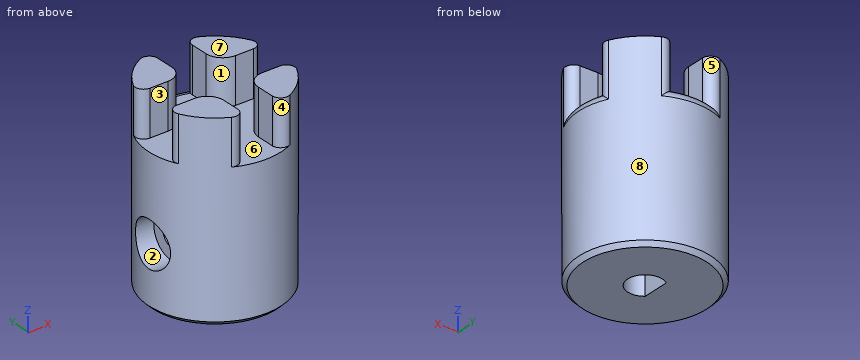
from build123d import *

# Parameters (mm, degrees)
SKETCH1_R           = 8
BOSS_EXTRUDE1_DEPTH = 23
CUT_EXTRUDE1_DEPTH  = 5.5
CHAMFER1_SIZE       = 0.5
FILLET1_R           = 1
SKETCH3_R           = 2.75
CUT_EXTRUDE2_DEPTH  = 15.5
SKETCH5_R           = 3.239790556
SKETCH5_R_2         = 1.3
BOSS_EXTRUDE2_DEPTH = 4


with BuildPart() as part:
    # Sketch1 → Boss-Extrude1 (new body)
    with BuildSketch(Plane.XY):
        Circle(SKETCH1_R)
        with BuildLine():
            Line((-1.3, 1.64924225), (-1.3, -1.64924225))
            ThreePointArc((-1.3, -1.64924225), (2.1, 0), (-1.3, 1.64924225))
        make_face(mode=Mode.SUBTRACT)
    extrude(amount=BOSS_EXTRUDE1_DEPTH)

    # Sketch2 → Cut-Extrude1 (cut)
    with BuildSketch(Plane.XY.offset(23)):
        with BuildLine():
            Line((4.1, 2.1), (9.874781321, 2.1))
            Line((9.874781321, 2.1), (9.874781321, -2.1))
            Line((9.874781321, -2.1), (4.1, -2.1))
            ThreePointArc((4.1, -2.1), (2.685786438, -2.685786438), (2.1, -4.1))
            Line((2.1, -4.1), (2.1, -8.269913673))
            Line((2.1, -8.269913673), (-2.1, -8.269913673))
            Line((-2.1, -8.269913673), (-2.1, -4.1))
            ThreePointArc((-2.1, -4.1), (-2.685786438, -2.685786438), (-4.1, -2.1))
            Line((-4.1, -2.1), (-9.874781321, -2.1))
            Line((-9.874781321, -2.1), (-9.874781321, 2.1))
            Line((-9.874781321, 2.1), (-4.1, 2.1))
            ThreePointArc((-4.1, 2.1), (-2.685786438, 2.685786438), (-2.1, 4.1))
            Line((-2.1, 4.1), (-2.1, 8.269913673))
            Line((-2.1, 8.269913673), (2.1, 8.269913673))
            Line((2.1, 8.269913673), (2.1, 4.1))
            ThreePointArc((2.1, 4.1), (2.685786438, 2.685786438), (4.1, 2.1))
        make_face()
    extrude(amount=-CUT_EXTRUDE1_DEPTH, mode=Mode.SUBTRACT)

    # Chamfer1
    chamfer1_edges = [part.edges().sort_by_distance(p)[0] for p in [
        (-8, 0, 0),
    ]]
    chamfer(chamfer1_edges, length=CHAMFER1_SIZE)

    # Fillet1
    # the kernel refuses this fillet: 1 mm, written as the material it takes off along each edge
    with BuildSketch(Plane(origin=(-7.719455939, 2.1, 26.857409903), x_dir=(0.35433001139154063, 0.9351204430592194, 0), z_dir=(0, 0, -1)), Plane(origin=(-2.1, -7.719455939, 26.857409903), x_dir=(-0.9351204430592192, 0.354330011391541, 0), z_dir=(0, 0, -1)), Plane(origin=(7.719455939, -2.1, 26.857409903), x_dir=(-0.354330011391541, -0.9351204430592192, 0), z_dir=(0, 0, -1)), Plane(origin=(2.1, 7.719455939, 26.857409903), x_dir=(0.935120443059219, -0.3543300113915411, 0), z_dir=(0, 0, -1))) as fillet1_piece_1:
        with BuildLine():
            CenterArc((1.446528713, 0.99533926), FILLET1_R, 159.247612079, 116.286320683)
            Line((0.51140827, 1.349669272), (0, 0))
            ThreePointArc((0, 0), (0.771481981, -0.037285918), (1.542963961, 0))
        make_face()
    extrude(amount=9.357409903, mode=Mode.SUBTRACT)
    with BuildSketch(Plane(origin=(-7.719455939, -2.1, 26.857409903), x_dir=(0.35433001139154124, -0.9351204430592192, 0), z_dir=(0, 0, -1)), Plane(origin=(2.1, -7.719455939, 26.857409903), x_dir=(0.935120443059219, 0.3543300113915412, 0), z_dir=(0, 0, -1)), Plane(origin=(7.719455939, 2.1, 26.857409903), x_dir=(-0.3543300113915409, 0.9351204430592193, 0), z_dir=(0, 0, -1)), Plane(origin=(-2.1, 7.719455939, 26.857409903), x_dir=(-0.935120443059219, -0.3543300113915412, 0), z_dir=(0, 0, -1))) as fillet1_piece_2:
        with BuildLine():
            CenterArc((1.446528713, -0.99533926), FILLET1_R, 84.466067237, 116.286320683)
            Line((0.51140827, -1.349669272), (0, 0))
            ThreePointArc((0, 0), (0.771481981, 0.037285918), (1.542963961, 0))
        make_face()
    extrude(amount=9.357409903, mode=Mode.SUBTRACT)
    with BuildSketch(Plane(origin=(0, 0, 17.5), x_dir=(1, 0, 0), z_dir=(0, 1, 0))) as fillet1_piece_3_section:
        with BuildLine():
            CenterArc((8 - FILLET1_R, FILLET1_R), FILLET1_R, 270, 90)
            Line((8 - FILLET1_R, 0), (8, 0))
            Line((8, 0), (8, FILLET1_R))
        make_face()
    fillet1_piece_3 = revolve(axis=Axis((0, 0, 17.5), (0, 0, -1)), revolution_arc=33.123591855, mode=Mode.PRIVATE)
    fillet1_piece_3 = split(fillet1_piece_3, bisect_by=Plane(origin=(7.676771465, -2.1, 17.273698774), z_dir=(0, 1, 0)), keep=Keep.TOP, mode=Mode.PRIVATE)
    add(fillet1_piece_3, mode=Mode.SUBTRACT)
    with BuildSketch(Plane(origin=(0, 0, 17.5), x_dir=(-0.5464558660226709, 0.8374879022943631, 0), z_dir=(-0.8374879022943631, -0.5464558660226709, 0))) as fillet1_piece_4_section:
        with BuildLine():
            CenterArc((8 - FILLET1_R, FILLET1_R), FILLET1_R, 270, 90)
            Line((8 - FILLET1_R, 0), (8, 0))
            Line((8, 0), (8, FILLET1_R))
        make_face()
    fillet1_piece_4 = revolve(axis=Axis((0, 0, 17.5), (0, 0, -1)), revolution_arc=66.248417342, mode=Mode.PRIVATE)
    fillet1_piece_4 = split(fillet1_piece_4, bisect_by=Plane(origin=(2.1, 7.676771683, 17.273698772), z_dir=(-1, 0, 0)), keep=Keep.TOP, mode=Mode.PRIVATE)
    fillet1_piece_4 = split(fillet1_piece_4, bisect_by=Plane(origin=(-2.1, 7.676771683, 17.273698772), z_dir=(1, 0, 0)), keep=Keep.TOP, mode=Mode.PRIVATE)
    add(fillet1_piece_4, mode=Mode.SUBTRACT)
    with BuildSketch(Plane(origin=(0, 0, 17.5), x_dir=(0.8374937851055057, 0.5464468500317786, 0), z_dir=(-0.5464468500317786, 0.8374937851055057, 0))) as fillet1_piece_5_section:
        with BuildLine():
            CenterArc((8 - FILLET1_R, FILLET1_R), FILLET1_R, 270, 90)
            Line((8 - FILLET1_R, 0), (8, 0))
            Line((8, 0), (8, FILLET1_R))
        make_face()
    fillet1_piece_5 = revolve(axis=Axis((0, 0, 17.5), (0, 0, -1)), revolution_arc=33.123591855, mode=Mode.PRIVATE)
    fillet1_piece_5 = split(fillet1_piece_5, bisect_by=Plane(origin=(7.676771942, 2.1, 17.273698679), z_dir=(0, -1, 0)), keep=Keep.TOP, mode=Mode.PRIVATE)
    add(fillet1_piece_5, mode=Mode.SUBTRACT)
    with BuildSketch(Plane(origin=(0, 0, 17.5), x_dir=(1, 0, 0), z_dir=(0, 1, 0))) as fillet1_piece_6a_section:
        with BuildLine():
            CenterArc((8 - FILLET1_R, FILLET1_R), FILLET1_R, 270, 90)
            Line((8 - FILLET1_R, 0), (8, 0))
            Line((8, 0), (8, FILLET1_R))
        make_face()
    fillet1_piece_6a = revolve(axis=Axis((0, 0, 17.5), (0, 0, -1)), revolution_arc=33.123591855, mode=Mode.PRIVATE)
    fillet1_piece_6a = split(fillet1_piece_6a, bisect_by=Plane(origin=(7.062995789, -2.1, 17.266816247), z_dir=(0, -1, 0)), keep=Keep.TOP, mode=Mode.PRIVATE)
    with BuildSketch(Plane(origin=(7.719455939, -2.1, 26.857409903), x_dir=(-0.354330011391541, -0.9351204430592192, 0), z_dir=(0, 0, -1))) as fillet1_piece_6b_section:
        with BuildLine():
            CenterArc((1.446528713, 0.99533926), FILLET1_R, 159.247612079, 116.286320683)
            Line((0.51140827, 1.349669272), (0, 0))
            ThreePointArc((0, 0), (0.771481981, -0.037285918), (1.542963961, 0))
        make_face()
    fillet1_piece_6b = extrude(amount=13.214819805, mode=Mode.PRIVATE)
    fillet1_piece_6b = split(fillet1_piece_6b, bisect_by=Plane(origin=(7.268798231, -2.449324776, 17.5), z_dir=(0, 0, -1)), keep=Keep.TOP, mode=Mode.PRIVATE)
    fillet1_piece_6 = fillet1_piece_6a & fillet1_piece_6b
    add(fillet1_piece_6, mode=Mode.SUBTRACT)
    with BuildSketch(Plane(origin=(0, 0, 17.5), x_dir=(0.8374937851055057, 0.5464468500317786, 0), z_dir=(-0.5464468500317786, 0.8374937851055057, 0))) as fillet1_piece_7a_section:
        with BuildLine():
            CenterArc((8 - FILLET1_R, FILLET1_R), FILLET1_R, 270, 90)
            Line((8 - FILLET1_R, 0), (8, 0))
            Line((8, 0), (8, FILLET1_R))
        make_face()
    fillet1_piece_7a = revolve(axis=Axis((0, 0, 17.5), (0, 0, -1)), revolution_arc=33.123591855, mode=Mode.PRIVATE)
    fillet1_piece_7a = split(fillet1_piece_7a, bisect_by=Plane(origin=(7.062995574, 2.1, 17.266816271), z_dir=(0, 1, 0)), keep=Keep.TOP, mode=Mode.PRIVATE)
    with BuildSketch(Plane(origin=(7.719455939, 2.1, 26.857409903), x_dir=(-0.3543300113915409, 0.9351204430592193, 0), z_dir=(0, 0, -1))) as fillet1_piece_7b_section:
        with BuildLine():
            CenterArc((1.446528713, -0.99533926), FILLET1_R, 84.466067237, 116.286320683)
            Line((0.51140827, -1.349669272), (0, 0))
            ThreePointArc((0, 0), (0.771481981, 0.037285918), (1.542963961, 0))
        make_face()
    fillet1_piece_7b = extrude(amount=13.214819805, mode=Mode.PRIVATE)
    fillet1_piece_7b = split(fillet1_piece_7b, bisect_by=Plane(origin=(7.268798231, 2.449324776, 17.5), z_dir=(0, 0, -1)), keep=Keep.TOP, mode=Mode.PRIVATE)
    fillet1_piece_7 = fillet1_piece_7a & fillet1_piece_7b
    add(fillet1_piece_7, mode=Mode.SUBTRACT)
    with BuildSketch(Plane(origin=(2.1, 7.719455939, 26.857409903), x_dir=(0.935120443059219, -0.3543300113915411, 0), z_dir=(0, 0, -1))) as fillet1_piece_8a_section:
        with BuildLine():
            CenterArc((1.446528713, 0.99533926), FILLET1_R, 159.247612079, 116.286320683)
            Line((0.51140827, 1.349669272), (0, 0))
            ThreePointArc((0, 0), (0.771481981, -0.037285918), (1.542963961, 0))
        make_face()
    fillet1_piece_8a = extrude(amount=13.214819805, mode=Mode.PRIVATE)
    fillet1_piece_8a = split(fillet1_piece_8a, bisect_by=Plane(origin=(2.449324776, 7.268798231, 17.5), z_dir=(0, 0, -1)), keep=Keep.TOP, mode=Mode.PRIVATE)
    with BuildSketch(Plane(origin=(0, 0, 17.5), x_dir=(-0.5464558660226709, 0.8374879022943631, 0), z_dir=(-0.8374879022943631, -0.5464558660226709, 0))) as fillet1_piece_8b_section:
        with BuildLine():
            CenterArc((8 - FILLET1_R, FILLET1_R), FILLET1_R, 270, 90)
            Line((8 - FILLET1_R, 0), (8, 0))
            Line((8, 0), (8, FILLET1_R))
        make_face()
    fillet1_piece_8b = revolve(axis=Axis((0, 0, 17.5), (0, 0, -1)), revolution_arc=66.248417342, mode=Mode.PRIVATE)
    fillet1_piece_8b = split(fillet1_piece_8b, bisect_by=Plane(origin=(2.1, 7.062976431, 17.266816363), z_dir=(1, 0, 0)), keep=Keep.TOP, mode=Mode.PRIVATE)
    fillet1_piece_8 = fillet1_piece_8a & fillet1_piece_8b
    add(fillet1_piece_8, mode=Mode.SUBTRACT)
    with BuildSketch(Plane(origin=(0, 0, 17.5), x_dir=(-0.5464558660226709, 0.8374879022943631, 0), z_dir=(-0.8374879022943631, -0.5464558660226709, 0))) as fillet1_piece_9a_section:
        with BuildLine():
            CenterArc((8 - FILLET1_R, FILLET1_R), FILLET1_R, 270, 90)
            Line((8 - FILLET1_R, 0), (8, 0))
            Line((8, 0), (8, FILLET1_R))
        make_face()
    fillet1_piece_9a = revolve(axis=Axis((0, 0, 17.5), (0, 0, -1)), revolution_arc=66.248417342, mode=Mode.PRIVATE)
    fillet1_piece_9a = split(fillet1_piece_9a, bisect_by=Plane(origin=(-2.1, 7.062976216, 17.266816386), z_dir=(-1, 0, 0)), keep=Keep.TOP, mode=Mode.PRIVATE)
    with BuildSketch(Plane(origin=(-2.1, 7.719455939, 26.857409903), x_dir=(-0.935120443059219, -0.3543300113915412, 0), z_dir=(0, 0, -1))) as fillet1_piece_9b_section:
        with BuildLine():
            CenterArc((1.446528713, -0.99533926), FILLET1_R, 84.466067237, 116.286320683)
            Line((0.51140827, -1.349669272), (0, 0))
            ThreePointArc((0, 0), (0.771481981, 0.037285918), (1.542963961, 0))
        make_face()
    fillet1_piece_9b = extrude(amount=13.214819805, mode=Mode.PRIVATE)
    fillet1_piece_9b = split(fillet1_piece_9b, bisect_by=Plane(origin=(-2.449324776, 7.268798231, 17.5), z_dir=(0, 0, -1)), keep=Keep.TOP, mode=Mode.PRIVATE)
    fillet1_piece_9 = fillet1_piece_9a & fillet1_piece_9b
    add(fillet1_piece_9, mode=Mode.SUBTRACT)

    # Sketch3 → Cut-Extrude2 (cut)
    with BuildSketch(Plane(origin=(-1.3, 0, 0), x_dir=(0, 0, -1), z_dir=(1, 0, 0))):
        with Locations(Location((-7.343789521, 0, 0), (0, 0, 36.850165711))):
            Circle(SKETCH3_R)
    extrude(amount=-CUT_EXTRUDE2_DEPTH, mode=Mode.SUBTRACT)

    # Sketch5 → Boss-Extrude2 (add)
    with BuildSketch(Plane(origin=(-1.3, 0, 0), x_dir=(0, 0, -1), z_dir=(1, 0, 0))):
        with Locations((-7.343789521, 0)):
            Circle(SKETCH5_R)
        with Locations((-7.343789521, 0)):
            Circle(SKETCH5_R_2, mode=Mode.SUBTRACT)
    extrude(amount=-BOSS_EXTRUDE2_DEPTH)


solid = part.part
Part model, mm, in its own coordinate system. Face numbers are marked on the shaded views. A direction names the side the tool comes from. Coordinates: 2 decimals unless noted, no trailing zeros. Loops run counter-clockwise (first coordinate to the right, second up) from the corner with the lowest first, then second, coordinate; pieces in that order, holes last. Notation, with made-up numbers: (38, 18.25) - (93, 18.25) arc R30 ccw to (93, 51.25) - close; hole circle Ø8 at (-23, 51). An arc over 180 degrees is marked (long way). Write each question's results on one line, items separated by ' | '. Start each with the question number.
Q1. Probe line 1 along X through (y, z) = (0, 13.5); line 2 along Z through (x, y) = (-6.7, 0); line 3 along X through (y, z) = (0, 9). List the from-to ranges inside material, lowest first.
Q2. Slice it at A-A on y = 0. Give the cut face in (x, z), and give its area (3 significant figures).
Q3. Which spindle directions (+Z, -Z, +X, -X, +Y, -Y) get a long thin tool onto all of the face, cutting with end or side? Do the marked faces 1, 2, 3 and 4. Say none if no direction does.
Q4. Two-plate mould, pull along Y, no slides. Class the marked faces 5, 6, 7 and 8: +Y half, -Y half, draft (parallel to the pull), parting line (faces both ways), or undercut.
Q5. Drop flat-ended pins along their axis: pin 1 Ø0.7 at (x, z) = (5, 21.5) entering from -Y; pin 2 Ø1.7 at (y, z) = (-5.5, 19.5) entering from -X; pin 3 Ø0.7 at (x, z) = (-5.5, 21.5) entering from -Y; pin 4 Ø6 at (y, z) = (-1, 10.5) entering from -X. Give the stop position or say it passes through.
Q6. Slice it at C-C on z = 19.75. Give the cut face in (x, y), and give its area (3 significant figures).
Q7. Slice it at B-B on x = 0. Give the cut face in (y, z), and give its area (3 significant figures).
Answer:
1) line 1: x = -8 to -1.3, 2.1 to 8 | line 2: z = 0 to 4.59, 10.09 to 17.5 | line 3: x = -5.3 to -1.3, 2.1 to 8
2) outline: (-8, 0.5) - (-7.5, 0) - (-1.3, 0) - (-1.3, 6.04) - (-5.3, 6.04) - (-5.3, 4.59) - (-8, 4.59) - close; (-8, 10.09) - (-5.3, 10.09) - (-5.3, 8.64) - (-1.3, 8.64) - (-1.3, 17.5) - (-8, 17.5) - close; (2.1, 0) - (7.5, 0) - (8, 0.5) - (8, 16.5) arc R1 ccw to (7, 17.5) - (2.1, 17.5) - close | area: 195 mm2
3) face 1: +Z | face 2: -X | face 3: +Z, +X, -X | face 4: +Z, -Y
4) face 5: +Y half | face 6: undercut | face 7: draft | face 8: parting line
5) pin 1: stops at y = -6.51 | pin 2: stops at x = -6.51 | pin 3: stops at y = -6.12 | pin 4: stops at x = -8
6) outline: (-7.17, -3.54) arc R8 ccw to (-3.54, -7.17) arc R1 ccw to (-2.1, -6.28) - (-2.1, -4.1) arc R2 ccw to (-4.1, -2.1) - (-6.28, -2.1) arc R1 ccw to start; (-7.17, 3.54) arc R1 ccw to (-6.28, 2.1) - (-4.1, 2.1) arc R2 ccw to (-2.1, 4.1) - (-2.1, 6.28) arc R1 ccw to (-3.54, 7.17) arc R8 ccw to start; (2.1, -6.28) arc R1 ccw to (3.54, -7.17) arc R8 ccw to (7.17, -3.54) arc R1 ccw to (6.28, -2.1) - (4.1, -2.1) arc R2 ccw to (2.1, -4.1) - close; (2.1, 4.1) arc R2 ccw to (4.1, 2.1) - (6.28, 2.1) arc R1 ccw to (7.17, 3.54) arc R8 ccw to (3.54, 7.17) arc R1 ccw to (2.1, 6.28) - close | area: 78.3 mm2
7) outline: (-8, 0.5) - (-7.5, 0) - (-2.1, 0) - (-2.1, 17.5) - (-8, 17.5) - close; (2.1, 0) - (7.5, 0) - (8, 0.5) - (8, 16.5) arc R1 ccw to (7, 17.5) - (2.1, 17.5) - close | area: 206 mm2
